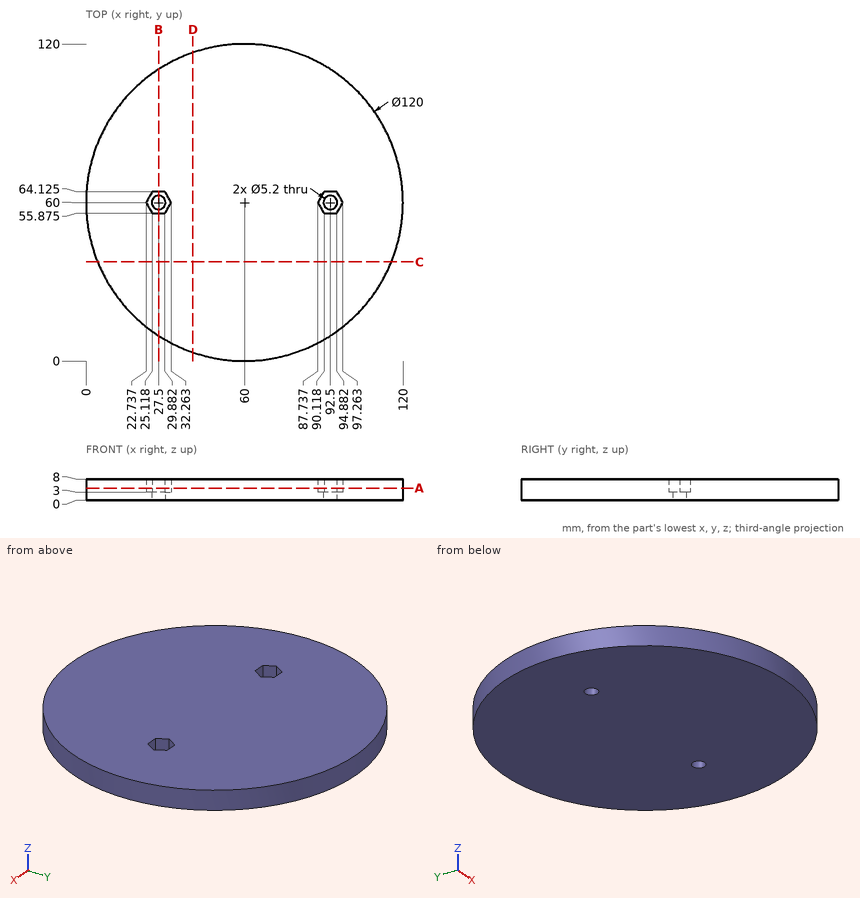
The figure shows three views and two pictorial views of one solid part (mm, origin at its lowest corner). Answer the questions. Round coordinates to 2 decimals unless told otherwise and drop trailing zeros. Write each loop counter-clockwise with the first axis right and the second up, starting at its lowest first coordinate (ties: lowest second). Pieces come first, ordered by that corner, then holes. Notation, with made-up numbers: M -8.75,83.25 L 1.25,83.25 A18 cw 1.25,117.25 Z; hole C 75,56.25 d5. An arc over 180 degrees is marked long. Use a Markdown table: item, result.
1) Flat-ended cylindrical pins translate along their axes: pin 1 (6 mm diameter, centred on x = 27.5, y = 60, fed in from +Z); pin 2 (2 mm diameter, centred on x = 24, z = 7, fed in from -Y) (1 decimal); pin 3 (1.4 mm diameter, centred on x = 26.5, z = 6.5, fed in from +Y). Find the tip coordinate at first contact, or state that the pin passes through.
Taken from the geometry:
| item | result |
|---|---|
| pin 1 | stops at z = 3 |
| pin 2 | stops at y = 11.3 |
| pin 3 | stops at y = 110.24 |
2) The part is cut by section B-B on x = 27.5. Give the vertices of the cut face in (y, z) (1 decimal).
Taken from the geometry:
| item | result |
|---|---|
| outline | M 9.6,0 L 57.4,0 L 57.4,3 L 55.9,3 L 55.9,8 L 9.6,8 Z; M 62.6,0 L 110.4,0 L 110.4,8 L 64.1,8 L 64.1,3 L 62.6,3 Z |
3) The part is cut by section A-A on z = 4.5. Give the vertices of the cut face in (x, y) (1 decimal), plus the area to 3 significant figures.
Taken from the geometry:
| item | result |
|---|---|
| outline | C 60,60 d120; hole M 22.7,60 L 25.1,55.9 L 29.9,55.9 L 32.3,60 L 29.9,64.1 L 25.1,64.1 Z; hole M 87.7,60 L 90.1,55.9 L 94.9,55.9 L 97.3,60 L 94.9,64.1 L 90.1,64.1 Z |
| area | 11,200 mm2 |
4) The part is cut by section C-C on y = 37.5. Give the vertices of the cut face in (x, z).
Taken from the geometry:
| item | result |
|---|---|
| outline | M 4.38,0 L 115.62,0 L 115.62,8 L 4.38,8 Z |
5) The part is cut by section D-D on x = 40.5. Give the vertices of the cut face in (y, z).
Taken from the geometry:
| item | result |
|---|---|
| outline | M 3.26,0 L 116.74,0 L 116.74,8 L 3.26,8 Z |
6) Consider line 1 (X direction, y = 63, z = 4.5) (1 decimal); line 2 (Y direction, x = 92.5, z = 0.75) (1 decimal); line 3 (Y direction, x = 8, z = 4) (1 decimal). Determine where each line is inside the solid, lowest interval first. Write a range as [from, to].
Taken from the geometry:
| item | result |
|---|---|
| line 1 | x = [0.1, 24.5], [30.5, 89.5], [95.5, 119.9] |
| line 2 | y = [9.6, 57.4], [62.6, 110.4] |
| line 3 | y = [30.1, 89.9] |
